Geometry check sheet. Reference: the model listing, model coordinates, mm. A direction names the side the tool comes from. Round coordinates to 2 decimals unless told otherwise and drop trailing zeros. Write each loop counter-clockwise with the first axis right and the second up, starting at its lowest first coordinate (ties: lowest second). Pieces come first, ordered by that corner, then holes.
Item 1: Cross-section at B-B (z = -1). Enter the section's corners in (x, y) (1 decimal).
Item 2: Draft check along Z on faces 1 (the face through (-1, 39.052, -5)), 2 (the face through (4, 1, -35.585)), 3 (the face through (-1, 37.148, -20)). Enter one of: pulls with the +Z half, pulls with the -Z half, needs draft (parallel to the pull), parting line crosses it, or undercut.
Item 3: Depth check by flat-ended pin: P1, Ø10, axis at x = -34, z = -21.5, coming from the +Y side; P2, Ø1.1, axis at x = -36, z = 38, coming from the +Y side; P3, Ø1.5, axis at x = 7, y = 1.5, coming from the -Z side; P4, Ø0.7, axis at y = 14.5, z = 38, coming from the -X side. Enter the tip coordinate at first touch or a pass-through.
Item 4: Access from +Z, -Z, +X, -X, +Y, -Y to the whole of each face (thin tool, end or side, straight path). Record for faces 4 (the face through (-1, 1.905, -20)), 5 (the face through (-1, 32.702, 0)), 6 (the face through (-1, 37.148, 20)).
Item 5: Scan lines: probe 1 along Y at (x, z) = (-48.5, -25.4); probe 2 along Z at (x, y) = (-9.5, 31.5); probe 3 along Y at (x, z) = (-46.5, 16). Record each from-to range of solid material in increasing order.
from build123d import *

# Parameters (mm, degrees)
SKETCH1_W                             = 104.4448
SKETCH1_H                             = 77.0128
BOSS_EXTRUDE1_DEPTH                   = 32.7025
SKETCH2_W                             = 104.4448
SKETCH2_H                             = 70.485
CUT_EXTRUDE1_DEPTH                    = 26.035
SKETCH3_W                             = 104.4448
SKETCH3_H                             = 77.0128
BOSS_EXTRUDE2_DEPTH                   = 6.35
SKETCH4_W                             = 19.05
SKETCH4_H                             = 2.921
CUT_EXTRUDE2_DEPTH                    = 20.32
SKETCH6_W                             = 14.1224
SKETCH6_H                             = 2.921
CUT_EXTRUDE3_DEPTH                    = 22.225
MIRROR2_COPY_1_SKETCH_W               = 19.05
MIRROR2_COPY_1_SKETCH_H               = 2.921
MIRROR2_COPY_1_DEPTH                  = 20.32
MIRROR2_COPY_2_SKETCH_W               = 14.1224
MIRROR2_COPY_2_SKETCH_H               = 2.921
MIRROR2_COPY_2_DEPTH                  = 22.225
SKETCH15_W                            = 2.921
SKETCH15_H                            = 3.175
CUT_EXTRUDE5_DEPTH                    = 106.669184434
FILLET2_R                             = 1.5875
FILLET2_OF_MIRROR6_R                  = 1.5875
F_56_0_0465_DIAMETER_HOLE1_AT_2_COUNT = 2
F_56_0_0465_DIAMETER_HOLE1_AT_2_PITCH = 10.16
F_56_0_0465_DIAMETER_HOLE1_AT_3_COUNT = 2
F_56_0_0465_DIAMETER_HOLE1_AT_3_PITCH = 20.32
F_56_0_0465_DIAMETER_HOLE1_AT_4_COUNT = 2
F_56_0_0465_DIAMETER_HOLE1_AT_4_PITCH = 37.428658221
F_56_0_0465_DIAMETER_HOLE1_AT_5_COUNT = 2
F_56_0_0465_DIAMETER_HOLE1_AT_5_PITCH = 33.033735124
F_56_0_0465_DIAMETER_HOLE1_AT_6_COUNT = 2
F_56_0_0465_DIAMETER_HOLE1_AT_6_PITCH = 31.4325
FILLET1_R                             = 1.5875
SKETCH13_W                            = 6.35
SKETCH13_H                            = 1.905
CUT_EXTRUDE4_DEPTH                    = 118.968456989
LPATTERN1_COUNT                       = 4
LPATTERN1_PITCH                       = 10.16
LPATTERN1_COL_COUNT                   = 4
LPATTERN1_COL_PITCH                   = 10.16


with BuildPart() as part:
    # Sketch1 → Boss-Extrude1 (new body)
    with BuildSketch(Plane(origin=(0, 0, 0), x_dir=(1, 0, 0), z_dir=(0, 1, 0))):
        Rectangle(SKETCH1_W, SKETCH1_H)
    extrude(amount=BOSS_EXTRUDE1_DEPTH)

    # Sketch2 → Cut-Extrude1 (cut)
    with BuildSketch(Plane(origin=(0, 32.7025, 0), x_dir=(1, 0, 0), z_dir=(0, 1, 0))):
        Rectangle(SKETCH2_W, SKETCH2_H)
    extrude(amount=-CUT_EXTRUDE1_DEPTH, mode=Mode.SUBTRACT)

    # Sketch3 → Boss-Extrude2 (add)
    with BuildSketch(Plane(origin=(0, 32.7025, 0), x_dir=(1, 0, 0), z_dir=(0, 1, 0))):
        Rectangle(SKETCH3_W, SKETCH3_H)
    extrude(amount=BOSS_EXTRUDE2_DEPTH)

    # Sketch4 → Cut-Extrude2 (cut)
    with BuildSketch(Plane(origin=(0, 39.0525, 0), x_dir=(1, 0, 0), z_dir=(0, 1, 0))):
        with Locations((42.6974, -37.0459)):
            Rectangle(SKETCH4_W, SKETCH4_H)
    cut_extrude2 = extrude(amount=-CUT_EXTRUDE2_DEPTH, mode=Mode.SUBTRACT)

    # Sketch6 → Cut-Extrude3 (cut)
    with BuildSketch(Plane.XZ):
        with Locations((45.1612, 37.0459)):
            Rectangle(SKETCH6_W, SKETCH6_H)
    cut_extrude3 = extrude(amount=-CUT_EXTRUDE3_DEPTH, mode=Mode.SUBTRACT)

    # Mirror1: Cut-Extrude2, Cut-Extrude3 across plane
    add(cut_extrude2.mirror(Plane.XY), mode=Mode.SUBTRACT)
    add(cut_extrude3.mirror(Plane.XY), mode=Mode.SUBTRACT)

    # Mirror2: Cut-Extrude2, Cut-Extrude3 across plane
    add(cut_extrude2.mirror(Plane(origin=(0, 0, 0), x_dir=(0, 0, 1), z_dir=(1, 0, 0))), mode=Mode.SUBTRACT)
    add(cut_extrude3.mirror(Plane(origin=(0, 0, 0), x_dir=(0, 0, 1), z_dir=(1, 0, 0))), mode=Mode.SUBTRACT)

    # Mirror2 copy 1 sketch → Mirror2 copy 1 (cut)
    with BuildSketch(Plane(origin=(0, 39.0525, 0), x_dir=(-1, 0, 0), z_dir=(0, 1, 0))):
        with Locations((42.6974, -37.0459)):
            Rectangle(MIRROR2_COPY_1_SKETCH_W, MIRROR2_COPY_1_SKETCH_H)
    extrude(amount=-MIRROR2_COPY_1_DEPTH, mode=Mode.SUBTRACT)

    # Mirror2 copy 2 sketch → Mirror2 copy 2 (cut)
    with BuildSketch(Plane(origin=(0, 0, 0), x_dir=(-1, 0, 0), z_dir=(0, -1, 0))):
        with Locations((45.1612, 37.0459)):
            Rectangle(MIRROR2_COPY_2_SKETCH_W, MIRROR2_COPY_2_SKETCH_H)
    extrude(amount=-MIRROR2_COPY_2_DEPTH, mode=Mode.SUBTRACT)

    # Sketch15 → Cut-Extrude5 (cut, through all)
    with BuildSketch(Plane(origin=(38.1, 0, 0), x_dir=(0, 0, -1), z_dir=(1, 0, 0))):
        with Locations((-37.0459, 1.5875)):
            Rectangle(SKETCH15_W, SKETCH15_H)
    cut_extrude5 = extrude(amount=-CUT_EXTRUDE5_DEPTH, mode=Mode.SUBTRACT)

    # Fillet2
    fillet2_edges = [part.edges().sort_by_distance(p)[0] for p in [
        (0, 3.175, 35.5854),
    ]]
    fillet(fillet2_edges, radius=FILLET2_R)

    # Mirror6: Cut-Extrude5 across plane
    add(cut_extrude5.mirror(Plane.XY), mode=Mode.SUBTRACT)

    # Fillet2 of Mirror6
    fillet2_of_mirror6_edges = [part.edges().sort_by_distance(p)[0] for p in [
        (0, 3.175, -35.5854),
    ]]
    fillet(fillet2_of_mirror6_edges, radius=FILLET2_OF_MIRROR6_R)

    # Sketch11 → #56 (0.0465) Diameter Hole1 (revolve, cut)
    with BuildSketch(Plane(origin=(-52.2224, 35.2425, -5.08), x_dir=(0, 0, 1), z_dir=(0, 1, 0))):
        Polygon((0, 0), (0, 9.879838239), (0.59055, 9.525), (0.59055, 0), align=None)
    f_56_0_0465_diameter_hole1 = revolve(axis=Axis((-58.5724, 35.2425, -5.08), (1, 0, 0)), mode=Mode.SUBTRACT)

    # #56 (0.0465) Diameter Hole1 at 2: #56 (0.0465) Diameter Hole1 ×2
    with Locations(*[(0, 0, -i * F_56_0_0465_DIAMETER_HOLE1_AT_2_PITCH) for i in range(1, F_56_0_0465_DIAMETER_HOLE1_AT_2_COUNT)]):
        add(f_56_0_0465_diameter_hole1, mode=Mode.SUBTRACT)

    # #56 (0.0465) Diameter Hole1 at 3: #56 (0.0465) Diameter Hole1 ×2
    with Locations(*[(0, 0, -i * F_56_0_0465_DIAMETER_HOLE1_AT_3_PITCH) for i in range(1, F_56_0_0465_DIAMETER_HOLE1_AT_3_COUNT)]):
        add(f_56_0_0465_diameter_hole1, mode=Mode.SUBTRACT)

    # #56 (0.0465) Diameter Hole1 at 4: #56 (0.0465) Diameter Hole1 ×2
    with Locations(*[Vector(0, -0.8397976709215131, -0.5428995044341098) * (i * F_56_0_0465_DIAMETER_HOLE1_AT_4_PITCH) for i in range(1, F_56_0_0465_DIAMETER_HOLE1_AT_4_COUNT)]):
        add(f_56_0_0465_diameter_hole1, mode=Mode.SUBTRACT)

    # #56 (0.0465) Diameter Hole1 at 5: #56 (0.0465) Diameter Hole1 ×2
    with Locations(*[Vector(0, -0.9515272760377812, -0.3075643720526165) * (i * F_56_0_0465_DIAMETER_HOLE1_AT_5_PITCH) for i in range(1, F_56_0_0465_DIAMETER_HOLE1_AT_5_COUNT)]):
        add(f_56_0_0465_diameter_hole1, mode=Mode.SUBTRACT)

    # #56 (0.0465) Diameter Hole1 at 6: #56 (0.0465) Diameter Hole1 ×2
    with Locations(*[(0, -i * F_56_0_0465_DIAMETER_HOLE1_AT_6_PITCH, 0) for i in range(1, F_56_0_0465_DIAMETER_HOLE1_AT_6_COUNT)]):
        add(f_56_0_0465_diameter_hole1, mode=Mode.SUBTRACT)

    # Mirror4: #56 (0.0465) Diameter Hole1 across plane
    add(f_56_0_0465_diameter_hole1.mirror(Plane.XY), mode=Mode.SUBTRACT)

    # Mirror4 copy 1 sketch → Mirror4 copy 1 (revolve, cut)
    with BuildSketch(Plane(origin=(-52.2224, 35.2425, 15.24), x_dir=(0, 0, -1), z_dir=(0, 1, 0))):
        Polygon((0, 0), (0, -9.879838239), (0.59055, -9.525), (0.59055, 0), align=None)
    revolve(axis=Axis((-58.5724, 35.2425, 15.24), (-1, 0, 0)), mode=Mode.SUBTRACT)

    # Mirror4 copy 2 sketch → Mirror4 copy 2 (revolve, cut)
    with BuildSketch(Plane(origin=(-52.2224, 35.2425, 25.4), x_dir=(0, 0, -1), z_dir=(0, 1, 0))):
        Polygon((0, 0), (0, -9.879838239), (0.59055, -9.525), (0.59055, 0), align=None)
    revolve(axis=Axis((-58.5724, 35.2425, 25.4), (-1, 0, 0)), mode=Mode.SUBTRACT)

    # Mirror4 copy 3 sketch → Mirror4 copy 3 (revolve, cut)
    with BuildSketch(Plane(origin=(-52.2224, 3.81, 25.4), x_dir=(0, 0, -1), z_dir=(0, 1, 0))):
        Polygon((0, 0), (0, -9.879838239), (0.59055, -9.525), (0.59055, 0), align=None)
    revolve(axis=Axis((-58.5724, 3.81, 25.4), (-1, 0, 0)), mode=Mode.SUBTRACT)

    # Mirror4 copy 4 sketch → Mirror4 copy 4 (revolve, cut)
    with BuildSketch(Plane(origin=(-52.2224, 3.81, 15.24), x_dir=(0, 0, -1), z_dir=(0, 1, 0))):
        Polygon((0, 0), (0, -9.879838239), (0.59055, -9.525), (0.59055, 0), align=None)
    revolve(axis=Axis((-58.5724, 3.81, 15.24), (-1, 0, 0)), mode=Mode.SUBTRACT)

    # Mirror4 copy 5 sketch → Mirror4 copy 5 (revolve, cut)
    with BuildSketch(Plane(origin=(-52.2224, 3.81, 5.08), x_dir=(0, 0, -1), z_dir=(0, 1, 0))):
        Polygon((0, 0), (0, -9.879838239), (0.59055, -9.525), (0.59055, 0), align=None)
    revolve(axis=Axis((-58.5724, 3.81, 5.08), (-1, 0, 0)), mode=Mode.SUBTRACT)

    # Mirror5: #56 (0.0465) Diameter Hole1 across plane
    add(f_56_0_0465_diameter_hole1.mirror(Plane(origin=(0, 0, 0), x_dir=(0, 0, 1), z_dir=(1, 0, 0))), mode=Mode.SUBTRACT)

    # Mirror5 copy 1 sketch → Mirror5 copy 1 (revolve, cut)
    with BuildSketch(Plane(origin=(52.2224, 35.2425, -15.24), x_dir=(0, 0, 1), z_dir=(0, 1, 0))):
        Polygon((0, 0), (0, -9.879838239), (0.59055, -9.525), (0.59055, 0), align=None)
    revolve(axis=Axis((58.5724, 35.2425, -15.24), (1, 0, 0)), mode=Mode.SUBTRACT)

    # Mirror5 copy 2 sketch → Mirror5 copy 2 (revolve, cut)
    with BuildSketch(Plane(origin=(52.2224, 35.2425, -25.4), x_dir=(0, 0, 1), z_dir=(0, 1, 0))):
        Polygon((0, 0), (0, -9.879838239), (0.59055, -9.525), (0.59055, 0), align=None)
    revolve(axis=Axis((58.5724, 35.2425, -25.4), (1, 0, 0)), mode=Mode.SUBTRACT)

    # Mirror5 copy 3 sketch → Mirror5 copy 3 (revolve, cut)
    with BuildSketch(Plane(origin=(52.2224, 3.81, -25.4), x_dir=(0, 0, 1), z_dir=(0, 1, 0))):
        Polygon((0, 0), (0, -9.879838239), (0.59055, -9.525), (0.59055, 0), align=None)
    revolve(axis=Axis((58.5724, 3.81, -25.4), (1, 0, 0)), mode=Mode.SUBTRACT)

    # Mirror5 copy 4 sketch → Mirror5 copy 4 (revolve, cut)
    with BuildSketch(Plane(origin=(52.2224, 3.81, -15.24), x_dir=(0, 0, 1), z_dir=(0, 1, 0))):
        Polygon((0, 0), (0, -9.879838239), (0.59055, -9.525), (0.59055, 0), align=None)
    revolve(axis=Axis((58.5724, 3.81, -15.24), (1, 0, 0)), mode=Mode.SUBTRACT)

    # Mirror5 copy 5 sketch → Mirror5 copy 5 (revolve, cut)
    with BuildSketch(Plane(origin=(52.2224, 3.81, -5.08), x_dir=(0, 0, 1), z_dir=(0, 1, 0))):
        Polygon((0, 0), (0, -9.879838239), (0.59055, -9.525), (0.59055, 0), align=None)
    revolve(axis=Axis((58.5724, 3.81, -5.08), (1, 0, 0)), mode=Mode.SUBTRACT)

    # Mirror5 copy 6 sketch → Mirror5 copy 6 (revolve, cut)
    with BuildSketch(Plane(origin=(52.2224, 35.2425, 5.08), x_dir=(0, 0, -1), z_dir=(0, 1, 0))):
        Polygon((0, 0), (0, 9.879838239), (0.59055, 9.525), (0.59055, 0), align=None)
    revolve(axis=Axis((58.5724, 35.2425, 5.08), (-1, 0, 0)), mode=Mode.SUBTRACT)

    # Mirror5 copy 7 sketch → Mirror5 copy 7 (revolve, cut)
    with BuildSketch(Plane(origin=(52.2224, 35.2425, 15.24), x_dir=(0, 0, -1), z_dir=(0, 1, 0))):
        Polygon((0, 0), (0, 9.879838239), (0.59055, 9.525), (0.59055, 0), align=None)
    revolve(axis=Axis((58.5724, 35.2425, 15.24), (-1, 0, 0)), mode=Mode.SUBTRACT)

    # Mirror5 copy 8 sketch → Mirror5 copy 8 (revolve, cut)
    with BuildSketch(Plane(origin=(52.2224, 35.2425, 25.4), x_dir=(0, 0, -1), z_dir=(0, 1, 0))):
        Polygon((0, 0), (0, 9.879838239), (0.59055, 9.525), (0.59055, 0), align=None)
    revolve(axis=Axis((58.5724, 35.2425, 25.4), (-1, 0, 0)), mode=Mode.SUBTRACT)

    # Mirror5 copy 9 sketch → Mirror5 copy 9 (revolve, cut)
    with BuildSketch(Plane(origin=(52.2224, 3.81, 25.4), x_dir=(0, 0, -1), z_dir=(0, 1, 0))):
        Polygon((0, 0), (0, 9.879838239), (0.59055, 9.525), (0.59055, 0), align=None)
    revolve(axis=Axis((58.5724, 3.81, 25.4), (-1, 0, 0)), mode=Mode.SUBTRACT)

    # Mirror5 copy 10 sketch → Mirror5 copy 10 (revolve, cut)
    with BuildSketch(Plane(origin=(52.2224, 3.81, 15.24), x_dir=(0, 0, -1), z_dir=(0, 1, 0))):
        Polygon((0, 0), (0, 9.879838239), (0.59055, 9.525), (0.59055, 0), align=None)
    revolve(axis=Axis((58.5724, 3.81, 15.24), (-1, 0, 0)), mode=Mode.SUBTRACT)

    # Mirror5 copy 11 sketch → Mirror5 copy 11 (revolve, cut)
    with BuildSketch(Plane(origin=(52.2224, 3.81, 5.08), x_dir=(0, 0, -1), z_dir=(0, 1, 0))):
        Polygon((0, 0), (0, 9.879838239), (0.59055, 9.525), (0.59055, 0), align=None)
    revolve(axis=Axis((58.5724, 3.81, 5.08), (-1, 0, 0)), mode=Mode.SUBTRACT)

    # Fillet1
    fillet1_edges = [part.edges().sort_by_distance(p)[0] for p in [
        (-33.1724, 18.7325, -37.0459),
        (-33.1724, 28.8925, -35.5854),
        (-35.6362, 18.7325, -35.5854),
        (-38.1, 10.16, -35.5854),
        (-33.1724, 28.8925, 35.5854),
        (-33.1724, 18.7325, 37.0459),
        (-35.6362, 18.7325, 35.5854),
        (-38.1, 10.16, 35.5854),
        (33.1724, 18.7325, 37.0459),
        (33.1724, 28.8925, 35.5854),
        (35.6362, 18.7325, 35.5854),
        (38.1, 10.16, 35.5854),
        (33.1724, 28.8925, -35.5854),
        (33.1724, 18.7325, -37.0459),
        (35.6362, 18.7325, -35.5854),
        (38.1, 10.16, -35.5854),
    ]]
    fillet(fillet1_edges, radius=FILLET1_R)

    # Sketch13 → Cut-Extrude4 (cut, through all)
    with BuildSketch(Plane.ZY.offset(52.2224)):
        with Locations((0, 38.1)):
            Rectangle(SKETCH13_W, SKETCH13_H)
        with Locations((0, 0.9525)):
            Rectangle(SKETCH13_W, SKETCH13_H)
    cut_extrude4 = extrude(amount=-CUT_EXTRUDE4_DEPTH, mode=Mode.SUBTRACT)

    # LPattern1: Cut-Extrude4 ×4
    with Locations(*[(0, 0, i * LPATTERN1_PITCH) for i in range(1, LPATTERN1_COUNT)]):
        add(cut_extrude4, mode=Mode.SUBTRACT)

    # LPattern1 col: Cut-Extrude4 ×4
    with Locations(*[(0, 0, -i * LPATTERN1_COL_PITCH) for i in range(1, LPATTERN1_COL_COUNT)]):
        add(cut_extrude4, mode=Mode.SUBTRACT)


solid = part.part
Resolved:
1. outline: (-52.2, 1.9) - (52.2, 1.9) - (52.2, 6.7) - (-52.2, 6.7) - close; (-52.2, 32.7) - (52.2, 32.7) - (52.2, 37.1) - (-52.2, 37.1) - close
2. face 1: needs draft
2. face 2: pulls with the -Z half
2. face 3: undercut
3. P1: stops at y = 39.05
3. P2: stops at y = 18.73
3. P3: stops at z = -35.73
3. P4: stops at x = -38.1
4. face 4: +X, -X, -Y
4. face 5: +X, -X
4. face 6: +X, -X, +Y
5. probe 1: y = 0 to 3.22, 4.4 to 6.67, 32.7 to 34.65, 35.83 to 39.05
5. probe 2: z = -38.51 to -35.24, 35.24 to 38.51
5. probe 3: y = 0 to 6.67, 32.7 to 39.05
